```python
from build123d import *

# Parameters (mm, degrees)
SKETCH1_W           = 180
SKETCH1_H           = 25
SKETCH1_R           = 7.5
BOSS_EXTRUDE1_DEPTH = 25
FILLET1_R           = 2.5
FILLET2_R           = 2.5


with BuildPart() as part:
    # Sketch1 → Boss-Extrude1 (new body)
    with BuildSketch(Plane.XY):
        with Locations((11.116046254, 73.038881715)):
            Rectangle(SKETCH1_W, SKETCH1_H)
        with Locations((-66.383953746, 73.038881715)):
            Circle(SKETCH1_R, mode=Mode.SUBTRACT)
        with Locations((88.616046254, 73.038881715)):
            Circle(SKETCH1_R, mode=Mode.SUBTRACT)
    extrude(amount=BOSS_EXTRUDE1_DEPTH)

    # Fillet1
    fillet1_edges = [part.edges().sort_by_distance(p)[0] for p in [
        (-78.883953746, 73.038881715, 25),
        (-78.883953746, 73.038881715, 0),
        (-78.883953746, 85.538881715, 12.5),
        (-78.883953746, 60.538881715, 12.5),
    ]]
    fillet(fillet1_edges, radius=FILLET1_R)

    # Fillet2
    fillet2_edges = [part.edges().sort_by_distance(p)[0] for p in [
        (101.116046254, 73.038881715, 25),
        (101.116046254, 73.038881715, 0),
        (101.116046254, 85.538881715, 12.5),
        (101.116046254, 60.538881715, 12.5),
    ]]
    fillet(fillet2_edges, radius=FILLET2_R)


solid = part.part
```
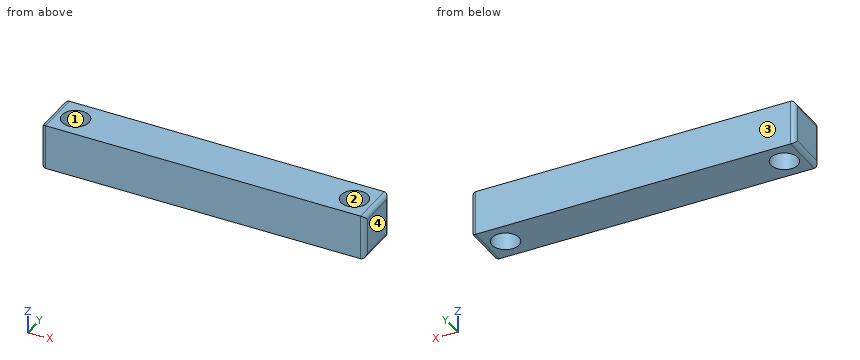
The model under review builds one solid part; all positions refer to its coordinate system, in mm. Face numbers are marked on the shaded views. Give positions to 0.01 mm unless a question says otherwise; leave off trailing zeros. Write each loop counter-clockwise with the first axis right and the second up, starting at its lowest first coordinate (ties: lowest second). Pieces come first, ordered by that corner, then holes.
(1) Consider section A-A, the plane y = 69.5. Give the boundary of the cut face in (x, z), and give its area (3 significant figures).
(2) Consider section D-D, the plane y = 76.75. Give the boundary of the cut face in (x, z).
(3) The part is to be moulded in two halves that separate along Y. For the marked faces 1, 2, 3 and 4, say which applies: released by +Y, released by -Y, zero draft, split by the parting line, or undercut.
(4) To check wall thickness, follow L1, parallel to X at y = 72.25, z = 8.25; L2, parallel to X at y = 73.5, z = 9.5; L3, parallel to Y at x = 93.5, z = 6.5. State the ranges of each line that lie inside material, in increasing order.
(5) Consider section C-C, the plane z = 17. Give the boundary of the cut face in (x, y), and give its area (3 significant figures).
(6) Consider section B-B, the plane x = 84. Give the boundary of the cut face in (y, z).
Returned:
1. outline: (-78.88, 2.5) arc R2.5 ccw to (-76.38, 0) - (-73, 0) - (-73, 25) - (-76.38, 25) arc R2.5 ccw to (-78.88, 22.5) - close; (-59.77, 0) - (82, 0) - (82, 25) - (-59.77, 25) - close; (95.23, 0) - (98.62, 0) arc R2.5 ccw to (101.12, 2.5) - (101.12, 22.5) arc R2.5 ccw to (98.62, 25) - (95.23, 25) - close
1. area: 3,830 mm2
2. outline: (-78.88, 2.5) arc R2.5 ccw to (-76.38, 0) - (-72.9, 0) - (-72.9, 25) - (-76.38, 25) arc R2.5 ccw to (-78.88, 22.5) - close; (-59.87, 0) - (82.1, 0) - (82.1, 25) - (-59.87, 25) - close; (95.13, 0) - (98.62, 0) arc R2.5 ccw to (101.12, 2.5) - (101.12, 22.5) arc R2.5 ccw to (98.62, 25) - (95.13, 25) - close
3. face 1: undercut
3. face 2: undercut
3. face 3: released by +Y
3. face 4: zero draft
4. L1: x = -78.88 to -73.84, -58.93 to 81.16, 96.07 to 101.12
4. L2: x = -78.88 to -73.87, -58.9 to 81.13, 96.1 to 101.12
4. L3: y = 60.54 to 67.35, 78.73 to 85.54
5. outline: (-78.88, 63.04) arc R2.5 ccw to (-76.38, 60.54) - (98.62, 60.54) arc R2.5 ccw to (101.12, 63.04) - (101.12, 83.04) arc R2.5 ccw to (98.62, 85.54) - (-76.38, 85.54) arc R2.5 ccw to (-78.88, 83.04) - close; hole circle Ø15 at (-66.38, 73.04); hole circle Ø15 at (88.62, 73.04)
5. area: 4,140 mm2
6. outline: (60.54, 0) - (67.13, 0) - (67.13, 25) - (60.54, 25) - close; (78.95, 0) - (85.54, 0) - (85.54, 25) - (78.95, 25) - close
